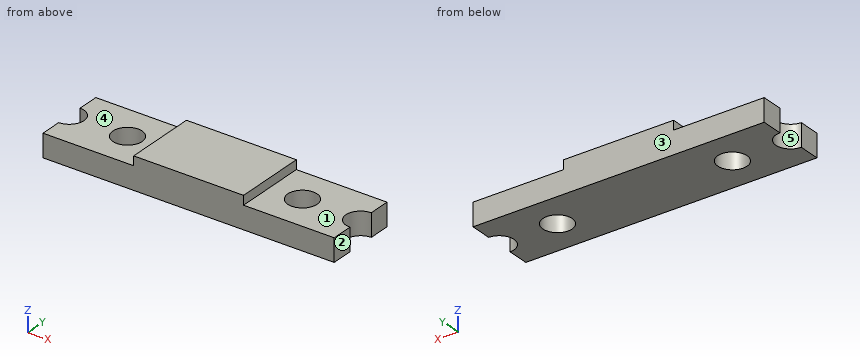
Autodesk Inventor part; units mm, degrees
ref_plane "YZ Plane" through (0, 0, 0) normal (1, 0, 0) x (0, 1, 0)
ref_plane "XZ Plane" through (0, 0, 0) normal (0, 1, 0) x (-1, 0, 0)
ref_plane "XY Plane" through (0, 0, 0) normal (0, 0, 1) x (1, 0, 0)
sketch "Sketch1" plane through (0, 0, 0) normal (0, 0, 1) x (1, 0, 0)
  line L0 (-15.9, -3.95) -> (15.9, -3.95)
  line L1 (15.9, -3.95) -> (15.9, 3.95)
  line L2 (15.9, 3.95) -> (-15.9, 3.95)
  line L3 (-15.9, 3.95) -> (-15.9, -3.95)
  line L4 (-15.9, -3.95) -> (15.9, 3.95) construction
  line L5 (15.9, -3.95) -> (-15.9, 3.95) construction
  line L6 (-15.9, 0) -> (15.9, 0) construction
  line L7 (0, 3.95) -> (0, -3.95) construction
  circle A0 centre (9.55, 0) radius 1.6
  arc A1 (15.9, 1.6) -> (15.9, -1.6) centre (15.9, 0) ccw
  circle A2 centre (-9.55, 0) radius 1.6
  arc A3 (-15.9, -1.6) -> (-15.9, 1.6) centre (-15.9, 0) ccw
  line L8 (6, 3.95) -> (6, -3.95)
  line L9 (-6, 3.95) -> (-6, -3.95)
  point P0 (0, 0)
  point P1 (-15.9, 1.6)
  point P2 (-15.9, -1.6)
  dimension "d0" = 31.8
  dimension "d1" = 7.9
  dimension "d2" = 3.2
  dimension "d3" = 19.1
  dimension "d4" = 12
extrude "Extrusion1" add sketch "Sketch1" along normal mid plane 2.5 contours L3 A3 L2 L9 L0 | L9 L2 L8 L0 | L8 L2 L1 A1 L0
extrude "Extrusion2" add sketch "Sketch1" along normal blind 2.25 contours L9 L2 L8 L0
properties part number "SC700-40kg"
The model under review builds one solid part; all positions refer to its coordinate system, in mm. Face numbers are marked on the shaded views. A direction names the side the tool comes from. Round coordinates to 2 decimals unless told otherwise and drop trailing zeros. Loops run counter-clockwise (first coordinate to the right, second up) from the corner with the lowest first, then second, coordinate; pieces in that order, holes last.
1) Tool access review of the marked faces 1 and 2: name each direction out of +Z, -Z, +X, -X, +Y, -Y from which nothing blocks a thin tool from reaching the whole face with its end or side.
Values follow:
face 1: +Z, +X, +Y, -Y
face 2: +Z, -Z, +X, +Y, -Y
2) The part is to be moulded in two halves that separate along Y. For the marked faces 3, 4 and 5, say which applies: pulls with the +Y half, pulls with the -Y half, needs draft (parallel to the pull), parting line crosses it, or undercut.
Values follow:
face 3: pulls with the +Y half
face 4: needs draft
face 5: undercut
3) Wall thickness on line 1 along Y through (x, z) = (9.55, 0.35); line 2 along X through (y, z) = (0.25, 0.8); line 3 along Z through (x, y) = (-12.5, -2): over which ranges is each line inside the solid? List them lowest first.
Values follow:
line 1: y = -3.95 to -1.6, 1.6 to 3.95
line 2: x = -14.32 to -11.13, -7.97 to 7.97, 11.13 to 14.32
line 3: z = -1.25 to 1.25
4) Consider section A-A on y = 0. State the section outline as (x, z) points.
Values follow:
outline: (-14.3, -1.25) - (-11.15, -1.25) - (-11.15, 1.25) - (-14.3, 1.25) - close; (-7.95, -1.25) - (7.95, -1.25) - (7.95, 1.25) - (6, 1.25) - (6, 2.25) - (-6, 2.25) - (-6, 1.25) - (-7.95, 1.25) - close; (11.15, -1.25) - (14.3, -1.25) - (14.3, 1.25) - (11.15, 1.25) - close
5) Consider section B-B on x = -9.55. State the section outline as (y, z) points, then the cut area to 4 significant figures.
Values follow:
outline: (-3.95, -1.25) - (-1.6, -1.25) - (-1.6, 1.25) - (-3.95, 1.25) - close; (1.6, -1.25) - (3.95, -1.25) - (3.95, 1.25) - (1.6, 1.25) - close
area: 11.75 mm2
6) Consider section D-D on y = -3. State the section outline as (x, z) points, then the cut area to 3 significant figures.
Values follow:
outline: (-15.9, -1.25) - (15.9, -1.25) - (15.9, 1.25) - (6, 1.25) - (6, 2.25) - (-6, 2.25) - (-6, 1.25) - (-15.9, 1.25) - close
area: 91.5 mm2
7) Consider section C-C on z = 0.8. State the section outline as (x, y) points.
Values follow:
outline: (-15.9, -3.95) - (15.9, -3.95) - (15.9, -1.6) arc R1.6 cw to (15.9, 1.6) - (15.9, 3.95) - (-15.9, 3.95) - (-15.9, 1.6) arc R1.6 cw to (-15.9, -1.6) - close; hole circle Ø3.2 at (-9.55, 0); hole circle Ø3.2 at (9.55, 0)
8) Clearance check with a flat-ended pin moving along its axis: P1, Ø2, axis at y = 0, z = 0, coming from the -X side. State where the tip first meets the part, or that it passes through.
Values follow:
P1: stops at x = -14.65
